Study the drawing (mm; zero at the part's minimum x, y, z) and answer. Give positions to 0.01 mm unless a question says otherwise; leave off trailing zeros. Write each loop counter-clockwise with the first axis right and the second up, starting at its lowest first coordinate (ties: lowest second). Pieces come first, ordered by that corner, then holes.
1) Find section B-B (x = 18). Determine the outline of the cut face in (y, z) (1 decimal).
2) Find section A-A (y = 4). Determine the outline of the cut face in (x, z), plus the area to 3 significant figures.
3) Find section D-D (z = 0.3). Count the separate pieces of the cut face and the enclosed holes in it.
4) Find section C-C (x = 25.5). Determine the outline of the cut face in (y, z) (1 decimal).
5) Straight lines are drawn through the part: probe 1 along Y at (x, z) = (4, 0.75) (1 decimal); probe 2 along Y at (x, z) = (24, 0.15) (1 decimal); probe 3 along Y at (x, z) = (18, 0.3) (1 decimal). For each, find the intervals that lie inside material, in ascending order.
6) Given pin 1 Ø2.5 at (x, y) = (25, 4) entering from +Z, flat-ended and moving along its own axis, determine where the tip first touches the part or whether it passes through.
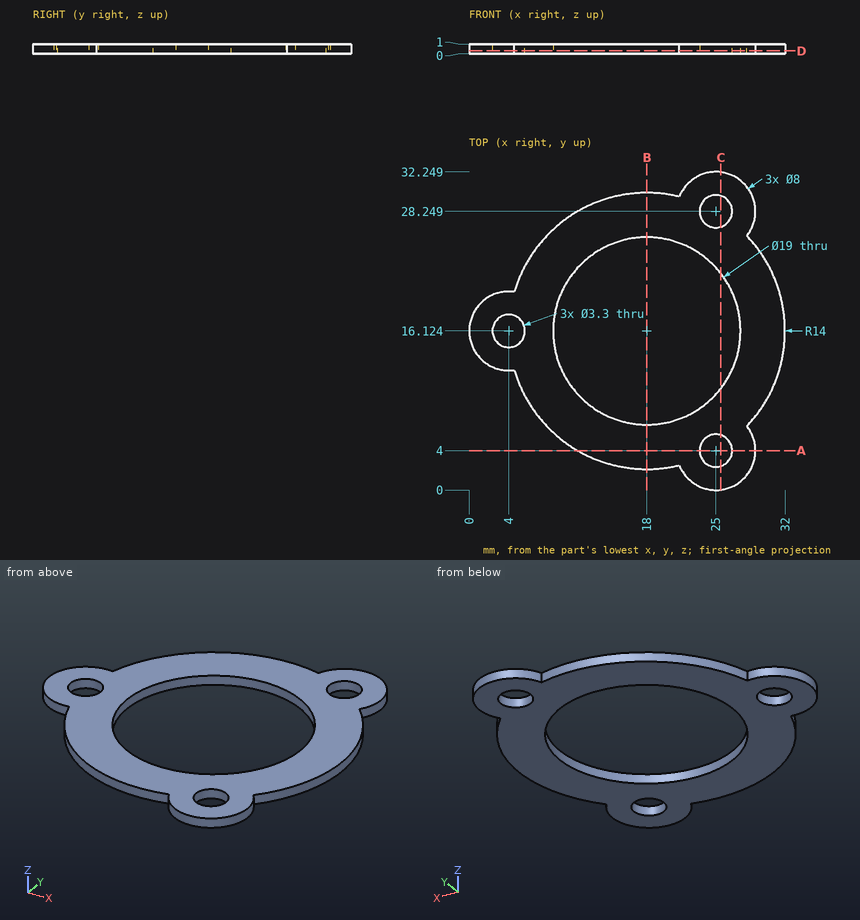
Results:
1. outline: (2.1, 0) - (6.6, 0) - (6.6, 1) - (2.1, 1) - close; (25.6, 0) - (30.1, 0) - (30.1, 1) - (25.6, 1) - close
2. outline: (11, 0) - (23.35, 0) - (23.35, 1) - (11, 1) - close; (26.65, 0) - (29, 0) - (29, 1) - (26.65, 1) - close
2. area: 14.7 mm2
3. separate pieces: 1
3. enclosed holes: 4
4. outline: (0, 0) - (2.4, 0) - (2.4, 1) - (0, 1) - close; (5.6, 0) - (10.3, 0) - (10.3, 1) - (5.6, 1) - close; (22, 0) - (26.7, 0) - (26.7, 1) - (22, 1) - close; (29.8, 0) - (32.2, 0) - (32.2, 1) - (29.8, 1) - close
5. probe 1: y = 12.1 to 14.5, 17.8 to 20.1
5. probe 2: y = 0.1 to 2.7, 5.3 to 8.8, 23.5 to 26.9, 29.6 to 32.1
5. probe 3: y = 2.1 to 6.6, 25.6 to 30.1
6. pin 1: passes through
